The figure shows three views and two pictorial views of one solid part (mm, origin at its lowest corner). Answer the questions. Round coordinates to 2 decimals unless told otherwise and drop trailing zeros. Order: outer loops, then holes, each group sorted by start corner. A loop starts at its lowest first (then second) coordinate and runs counter-clockwise, first axis right, second up. Notation, with made-up numbers: (52.25, -37) - (62.25, -37) arc R27 ccw to (62.25, -20) - close; hole circle Ø5 at (56, 48). An arc over 180 degrees is marked (long way). Answer as a JSON object with one key per item and string values. Group by question number.
Q1. Given pin 1 Ø8 at (y, z) = (15, 11) entering from -X; pin 2 Ø12 at (x, z) = (12, 25) entering from +Y; pin 3 Ø12 at (x, y) = (16.5, 24.5) entering from -Z; pin 4 Ø4 at (x, z) = (14, 15.5) entering from +Y, each flat-ended and moving along its own axis, determine where each tip first touches the part or whether it passes through.
Q2. Consider line 1 (Y direction, x = 4.25, z = 15); line 2 (Y direction, x = 18.8, z = 15); line 3 (X direction, y = 3, z = 19.5). Determine where each line is inside the solid, lowest interval first.
Q3. A cutting plane is placed at D-D on z = 26.5. Determine the outline of the cut face in (x, y), and give its area (3 significant figures).
Q4. The mould has two halves that part along Y. Classify the marked faces 1, 2 and 3: pulls with the +Y half, pulls with the -Y half, needs draft (parallel to the pull), parting line crosses it, or undercut.
Q5. A cutting plane is placed at A-A on z = 15. Determine the outline of the cut face in (x, y).
Q6. A cutting plane is placed at C-C on x = 10.25. Determine the outline of the cut face in (y, z).
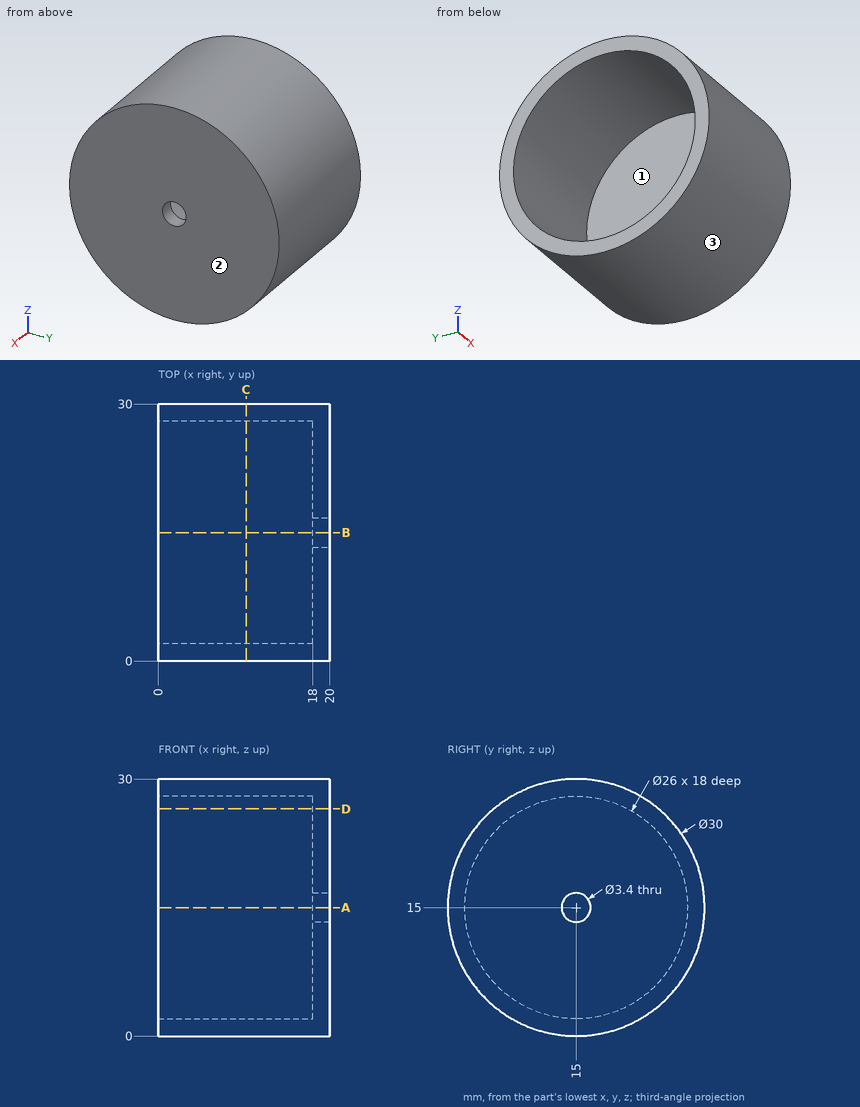
Result set:
{
 "1": {"pin 1": "stops at x = 18", "pin 2": "stops at y = 29.46", "pin 3": "stops at z = 0.41", "pin 4": "stops at y = 30"},
 "2": {"line 1": "y = 0 to 2, 28 to 30", "line 2": "y = 0 to 13.3, 16.7 to 30", "line 3": "x = 18 to 20"},
 "3": {"outline": "(0, 5.37) - (20, 5.37) - (20, 24.63) - (0, 24.63) - (0, 21.06) - (18, 21.06) - (18, 8.94) - (0, 8.94) - close", "area": "167 mm²"},
 "4": {"face 1": "undercut", "face 2": "needs draft", "face 3": "parting line crosses it"},
 "5": {"outline": "(0, 0) - (20, 0) - (20, 13.3) - (18, 13.3) - (18, 2) - (0, 2) - close; (0, 28) - (18, 28) - (18, 16.7) - (20, 16.7) - (20, 30) - (0, 30) - close"},
 "6": {"outline": "circle Ø30 at (15, 15); hole circle Ø26 at (15, 15)"}
}
